Part model, mm, in its own coordinate system. A direction names the side the tool comes from. Round coordinates to 2 decimals unless told otherwise and drop trailing zeros. Loops run counter-clockwise (first coordinate to the right, second up) from the corner with the lowest first, then second, coordinate; pieces in that order, holes last. Notation, with made-up numbers: (82.25, 81) - (95.25, 81) arc R10 cw to (95.25, 94) - close; hole circle Ø10 at (-38, 24). An arc over 180 degrees is marked (long way). Write each question's results on one line, items separated by ' | '. Start each with the question number.
(1) Cut at A-A, the plane y = 9. List the corners of the cut face in (x, z), then the cut area to 3 significant figures.
(2) Flat gauge pins, fed straight in: P1, Ø1.5, axis at y = 13, z = -6, coming from the -X side; P2, Ø10.5, axis at x = 9, y = 6.5, coming from the -Z side; P3, Ø11.5, axis at x = -0.05, z = -2.83, coming from the +Y side. Where does each tip first touch, or does it go through?
(3) Mould opens along X. For faces 1 (the face through (-10, 6, -6.333)), 2 (the face through (-4, 0, 2)), 3 (the face through (-13.44, 10.86, -20.29)) say: released by +X, released by -X, zero draft, split by the parting line, or undercut.
(4) Cut at D-D, the plane y = 18. List the corners of the cut face in (x, z), then the cut area to 3 significant figures.
(5) Tool access for faces 4 (the face through (11, 22, 8)), 5 (the face through (4.481, 5.916, -7.494)), 6 (the face through (2.211, 11.014, -6.724)): list every direction of +Z, -Z, +X, -X, +Y, -Y with a clear straight run to the whole face (end or side of a thin tool).
(6) Drill centre lines: L1, parallel to Z at x = 11, y = 2.5; L2, parallel to X at y = 8.5, z = -15.5; L3, parallel to Z at x = 0, y = 5.5. Where is each one in solid material? Low to high.
(7) Cut at B-B, the plane x = 13. Give the number of separate pieces and of enclosed holes in the cut face, then the cut area to 3 significant figures.
from build123d import *

# Parameters (mm, degrees)
SKETCH1_R           = 22
SKETCH1_R_2         = 15.236020103
BOSS_EXTRUDE2_DEPTH = 22
SKETCH3_R           = 1.5
BOSS_EXTRUDE3_DEPTH = 12
SKETCH4_R           = 4.990818698
CUT_EXTRUDE1_DEPTH  = 6
CUT_EXTRUDE2_DEPTH  = 2
FILLET1_R           = 1
FILLET2_R           = 1


with BuildPart() as part:
    # Sketch1 → Boss-Extrude2 (new body)
    with BuildSketch(Plane(origin=(0, 0, 0), x_dir=(1, 0, 0), z_dir=(0, 1, 0))):
        with Locations(Location((-0.049514064, 2.832612422, 0), (0, 0, 270))):
            Circle(SKETCH1_R)
        with Locations(Location((-0.049514064, 2.832612422, 0), (0, 0, 270))):
            Circle(SKETCH1_R_2, mode=Mode.SUBTRACT)
    extrude(amount=BOSS_EXTRUDE2_DEPTH)


with BuildPart() as boss_extrude3_tool:
    # Sketch3 → Boss-Extrude3 (new body)
    with BuildSketch(Plane(origin=(0, 0, 0), x_dir=(-1, 0, 0), z_dir=(0, -1, 0))):
        with BuildLine():
            Line((-3.328678892, 17.689399127), (-3.328678892, 8.385792362))
            ThreePointArc((-3.328678892, 8.385792362), (-4.495647669, 7.479277859), (-5.427711213, 6.332612162))
            Line((-5.427711213, 6.332612162), (-14.77904958, 6.332612162))
            ThreePointArc((-14.77904958, 6.332612162), (-15.186505741, 2.832612162), (-14.77904958, -0.667387838))
            Line((-14.77904958, -0.667387838), (-5.427711213, -0.667387838))
            ThreePointArc((-5.427711213, -0.667387838), (-4.495647669, -1.814053536), (-3.328678892, -2.720568038))
            Line((-3.328678892, -2.720568038), (-3.328678892, -12.024174803))
            ThreePointArc((-3.328678892, -12.024174803), (0.174668323, -12.402893904), (3.671321108, -11.966672432))
            Line((3.671321108, -11.966672432), (3.671321108, -2.564842414))
            ThreePointArc((3.671321108, -2.564842414), (4.696898655, -1.711815111), (5.526739937, -0.667387838))
            Line((5.526739937, -0.667387838), (14.878078304, -0.667387838))
            ThreePointArc((14.878078304, -0.667387838), (15.183327611, 1.070793462), (15.285534465, 2.832612162))
            ThreePointArc((15.285534465, 2.832612162), (15.183327611, 4.594430862), (14.878078304, 6.332612162))
            Line((14.878078304, 6.332612162), (5.526739937, 6.332612162))
            ThreePointArc((5.526739937, 6.332612162), (4.696898655, 7.377039435), (3.671321108, 8.230066738))
            Line((3.671321108, 8.230066738), (3.671321108, 17.631896755))
            ThreePointArc((3.671321108, 17.631896755), (0.174668323, 18.068118227), (-3.328678892, 17.689399127))
        make_face()
        with Locations(Location((0.049514362, 2.832612162, 0), (0, 0, 90))):
            Circle(SKETCH3_R, mode=Mode.SUBTRACT)
    extrude(amount=-BOSS_EXTRUDE3_DEPTH)


with BuildPart() as part_1:
    add(part.part)


with BuildPart() as part_2:
    # Boss-Extrude3: joined with boss_extrude3_tool
    add(part_1.part.fuse(boss_extrude3_tool.part, tol=0.00001))

    # Sketch4 → Cut-Extrude1 (cut)
    with BuildSketch(Plane(origin=(0, 0, 0), x_dir=(-1, 0, 0), z_dir=(0, -1, 0))):
        with Locations(Location((0.049514362, 2.832612162, 0), (0, 0, 90))):
            Circle(SKETCH4_R)
    extrude(amount=-CUT_EXTRUDE1_DEPTH, mode=Mode.SUBTRACT)

    # Sketch5 → Cut-Extrude2 (cut)
    with BuildSketch(Plane(origin=(0, 12, 0), x_dir=(1, 0, 0), z_dir=(0, 1, 0))):
        Polygon((-4.56347244, 5.406360618), (-4.535424574, 0.210283895), (-0.021466198, -2.363464302), (4.464444311, 0.258864225), (4.436396445, 5.454940948), (-0.077561931, 8.028689145), align=None)
    extrude(amount=-CUT_EXTRUDE2_DEPTH, mode=Mode.SUBTRACT)

    # Fillet1
    fillet1_edges = [part_2.edges().sort_by_distance(p)[0] for p in [
        (-0.049514064, 22, -24.832612422),
    ]]
    fillet(fillet1_edges, radius=FILLET1_R)

    # Fillet2
    fillet2_edges = [part_2.edges().sort_by_distance(p)[0] for p in [
        (-0.049514064, 0, -24.832612422),
    ]]
    fillet(fillet2_edges, radius=FILLET2_R)


solid = part_2.part
A:
1) outline: circle Ø44 at (-0.05, -2.83); hole (-14.88, -6.33) arc R15.24 ccw to (-3.67, -17.63) - (-3.67, -8.23) arc R6.5 cw to (-5.53, -6.33) - close; hole (-14.88, 0.67) - (-5.53, 0.67) arc R6.5 cw to (-3.67, 2.56) - (-3.67, 11.97) arc R15.24 ccw to start; hole circle Ø3 at (-0.05, -2.83); hole (3.33, -17.69) arc R15.24 ccw to (14.78, -6.33) - (5.43, -6.33) arc R6.5 cw to (3.33, -8.39) - close; hole (3.33, 2.72) arc R6.5 cw to (5.43, 0.67) - (14.78, 0.67) arc R15.24 ccw to (3.33, 12.02) - close | area: 1,170 mm2
2) P1: x = -21.92 | P2: z = -24.5 | P3: y = 12
3) face 1: undercut | face 2: zero draft | face 3: split by the parting line
4) outline: circle Ø44 at (-0.05, -2.83); hole circle Ø30.47 at (-0.05, -2.83) | area: 791 mm2
5) face 4: +Z, -Z, +X, -X, +Y | face 5: +Y, -Y | face 6: +Y
6) L1: -21.86 to -13.32, -6.33 to 0.67, 7.66 to 16.19 | L2: -18.04 to -8.52, -3.67 to 3.33, 8.42 to 17.94 | L3: -24.83 to -7.82, 2.16 to 19.17
7) separate pieces: 3 | enclosed holes: 0 | area: 516 mm2
